CAD build for the part. Positions are in the model's coordinates, mm. Coordinates: 2 decimals unless noted, no trailing zeros. Write each loop counter-clockwise with the first axis right and the second up, starting at its lowest first coordinate (ties: lowest second). Pieces come first, ordered by that corner, then holes. Notation, with made-up numbers: M -32.5,59 L 23.5,59 A27 ccw 23.5,92 Z; hole C 72,45.25 d10. An arc over 180 degrees is marked long. Answer as CSV lines item,"result". Start each with the question number.
```python
from build123d import *

# Parameters (mm, degrees)
F0_W     = 104
F0_H     = 15
F0_R     = 5
F0_R_2   = 2
F1_DEPTH = 10
F2_R     = 0.75
F3_DEPTH = 25


with BuildPart() as f1:
    # F0 (on Top) → F1 (new body)
    with BuildSketch(Plane.XY):
        Rectangle(F0_W, F0_H)
        with Locations((-37, 0)):
            Circle(F0_R, mode=Mode.SUBTRACT)
        with Locations((-25, 0)):
            Circle(F0_R_2, mode=Mode.SUBTRACT)
        with Locations((25, 0)):
            Circle(F0_R_2, mode=Mode.SUBTRACT)
        with Locations((37, 0)):
            Circle(F0_R, mode=Mode.SUBTRACT)
    extrude(amount=F1_DEPTH)

    # F2 (on face) → F3 (cut)
    with BuildSketch(Plane.XZ.offset(7.5)):
        with Locations((-43.5, 5.666667)):
            Circle(F2_R)
        with Locations((-31, 5.666667)):
            Circle(F2_R)
        with Locations((-18.5, 5.666667)):
            Circle(F2_R)
        with Locations((-6, 5.666667)):
            Circle(F2_R)
        with Locations((6.5, 5.666667)):
            Circle(F2_R)
        with Locations((19, 5.666667)):
            Circle(F2_R)
        with Locations((31.5, 5.666667)):
            Circle(F2_R)
        with Locations((44, 5.666667)):
            Circle(F2_R)
    extrude(amount=-F3_DEPTH, mode=Mode.SUBTRACT)


solid = f1.part
```
1) Band-saw the part on C-C, the plane y = 0. State how many separate pieces and enclosed holes the cut face has, plus the area to 3 significant figures.
2) Band-saw the part on D-D, the plane x = 37. List the corners of the cut face in (y, z), plus the area to 3 significant figures.
3) Band-saw the part on A-A, the plane x = 25. List the corners of the cut face in (y, z).
4) Probe L1, parallel to X at y = -0.25, z = 7.75; L2, parallel to X at y = 3.25, z = 1.5; L3, parallel to X at y = 0.5, z = 0.75. List the from-to ranges inside material, lowest first. Write a range as [from, to].
5) Pin check, flat tips, straight feed: P1, Ø2, axis at x = -31, z = 5.67, coming from the -Y side; P2, Ø1.4, axis at x = -18.5, z = 5.67, coming from the -Y side. Stop position of each tip, or through.
6) Band-saw the part on B-B, the plane z = 8.75. List the corners of the cut face in (x, y), plus the area to 3 significant figures.
7) Two-plate mould, pull along Y, no slides. Class faces 1 (the cylindrical face through (23, 0, 5)), 2 (the flat face through (-1, -7.5, 5)), 3 (the flat face through (-52, 0, 5)): pulls with the +Y half, pulls with the -Y half, needs draft (parallel to the pull), parting line crosses it, or undercut.
Result sheet:
1,separate pieces,"5"
1,enclosed holes,"7"
1,area,"746 mm²"
2,outline,"M -7.5,0 L -5,0 L -5,10 L -7.5,10 Z; M 5,0 L 7.5,0 L 7.5,10 L 5,10 Z"
2,area,"50.0 mm²"
3,outline,"M -7.5,0 L -2,0 L -2,10 L -7.5,10 Z; M 2,0 L 7.5,0 L 7.5,10 L 2,10 Z"
4,L1,"x = [-52, -41.99], [-32.01, -26.98], [-23.02, 23.02], [26.98, 32.01], [41.99, 52]"
4,L2,"x = [-52, -40.8], [-33.2, 33.2], [40.8, 52]"
4,L3,"x = [-52, -41.97], [-32.03, -26.94], [-23.06, 23.06], [26.94, 32.03], [41.97, 52]"
5,P1,"stops at y = -7.5"
5,P2,"passes through"
6,outline,"M -52,-7.5 L 52,-7.5 L 52,7.5 L -52,7.5 Z; hole C -37,0 d10; hole C -25,0 d4; hole C 25,0 d4; hole C 37,0 d10"
6,area,"1,380 mm²"
7,face 1,"undercut"
7,face 2,"pulls with the -Y half"
7,face 3,"needs draft"
